from build123d import *

# Parameters (mm, degrees)
BOSS_EXTRUDE1_DEPTH = 40
BOSS_EXTRUDE3_DEPTH = 2.35
BOSS_EXTRUDE4_DEPTH = 2.7
SKETCH7_R           = 5
BOSS_EXTRUDE5_DEPTH = 1
SKETCH8_R           = 2.5
BOSS_EXTRUDE6_DEPTH = 4.6
BOSS_EXTRUDE7_DEPTH = 0.5


with BuildPart() as part:
    # Sketch1 → Boss-Extrude1 (new body)
    with BuildSketch(Plane.XY):
        with BuildLine():
            Line((1.27, 0), (18.68, 0))
            ThreePointArc((18.68, 0), (19.578025612, 0.371974388), (19.95, 1.27))
            Line((19.95, 1.27), (19.95, 36.4))
            Line((19.95, 36.4), (0, 36.4))
            Line((0, 36.4), (0, 1.27))
            ThreePointArc((0, 1.27), (0.371974388, 0.371974388), (1.27, 0))
        make_face()
    extrude(amount=BOSS_EXTRUDE1_DEPTH)

    # Sketch5 → Boss-Extrude3 (add)
    with BuildSketch(Plane(origin=(0, 28, 0), x_dir=(-1, 0, 0), z_dir=(0, -1, 0))):
        with BuildLine():
            Line((0, 0), (0, 7))
            Line((0, 7), (-3.470401751, 7))
            Line((-3.470401751, 7), (-2.98203275, 5.390690104))
            ThreePointArc((-2.98203275, 5.390690104), (-4.95, 2.05), (-6.91796725, 5.390690104))
            Line((-6.91796725, 5.390690104), (-6.429598249, 7))
            Line((-6.429598249, 7), (-13.370401751, 7))
            Line((-13.370401751, 7), (-12.88203275, 5.390690104))
            ThreePointArc((-12.88203275, 5.390690104), (-14.85, 2.05), (-16.81796725, 5.390690104))
            Line((-16.81796725, 5.390690104), (-16.329598249, 7))
            Line((-16.329598249, 7), (-19.8, 7))
            Line((-19.8, 7), (-19.8, 0))
            Line((-19.8, 0), (0, 0))
        make_face()
        with BuildLine():
            Line((-16.329598249, -47), (-16.81796725, -45.390690104))
            ThreePointArc((-16.81796725, -45.390690104), (-14.85, -42.05), (-12.88203275, -45.390690104))
            Line((-12.88203275, -45.390690104), (-13.370401751, -47))
            Line((-13.370401751, -47), (-6.429598249, -47))
            Line((-6.429598249, -47), (-6.91796725, -45.390690104))
            ThreePointArc((-6.91796725, -45.390690104), (-4.95, -42.05), (-2.98203275, -45.390690104))
            Line((-2.98203275, -45.390690104), (-3.470401751, -47))
            Line((-3.470401751, -47), (0, -47))
            Line((0, -47), (0, -40))
            Line((0, -40), (-19.8, -40))
            Line((-19.8, -40), (-19.8, -47))
            Line((-19.8, -47), (-16.329598249, -47))
        make_face()
    extrude(amount=-BOSS_EXTRUDE3_DEPTH)

    # Sketch6 → Boss-Extrude4 (add)
    with BuildSketch(Plane(origin=(0, 36.4, 0), x_dir=(1, 0, 0), z_dir=(0, 1, 0))):
        with BuildLine():
            Line((19.95, -3.7), (19.95, -40))
            Line((19.95, -40), (0, -40))
            Line((0, -40), (0, -3.7))
            Line((0, -3.7), (8.380131585, -3.7))
            ThreePointArc((8.380131585, -3.7), (9.9, -3), (11.419868415, -3.7))
            Line((11.419868415, -3.7), (19.95, -3.7))
        make_face()
    extrude(amount=BOSS_EXTRUDE4_DEPTH)

    # Sketch7 → Boss-Extrude5 (add)
    with BuildSketch(Plane(origin=(0, 39.1, 0), x_dir=(1, 0, 0), z_dir=(0, 1, 0))):
        with Locations((9.95, -30)):
            Circle(SKETCH7_R)
    extrude(amount=BOSS_EXTRUDE5_DEPTH)

    # Sketch8 → Boss-Extrude6 (add)
    with BuildSketch(Plane(origin=(0, 40.1, 0), x_dir=(1, 0, 0), z_dir=(0, 1, 0))):
        with Locations((9.95, -30)):
            Circle(SKETCH8_R)
    extrude(amount=BOSS_EXTRUDE6_DEPTH)

    # Sketch9 → Boss-Extrude7 (add, symmetric)
    with BuildSketch(Plane.ZY.offset(-9.9)):
        Polygon((47, 30.35), (40, 34.1), (40, 30.35), align=None)
    extrude(amount=BOSS_EXTRUDE7_DEPTH, both=True)


solid = part.part
Verification items for the finished model (mm, model axes). A direction names the side the tool comes from. Give positions to 0.01 mm unless a question says otherwise; leave off trailing zeros. Order: outer loops, then holes, each group sorted by start corner. A loop starts at its lowest first (then second) coordinate and runs counter-clockwise, first axis right, second up. Notation, with made-up numbers: M 70.25,36 L 80.25,36 A14 ccw 80.25,63 Z; hole C 44.5,-0.75 d2. An arc over 180 degrees is marked long. Answer as a JSON object with one key per item and string values. Group by question number.
1) Access from +Z, -Z, +X, -X, +Y, -Y to the whole of each face (thin tool, end or side, straight path). Record for faces 1 (the face through (4.8, 30.35, 41.9)), 2 (the face through (16.58, 29.16, -6.18)), 3 (the face through (10.4, 31, 42)).
2) Cross-section at C-C (y = 13.5). Enter the section's corners in (x, z).
3) Cross-section at D-D (z = 44.3). Enter the section's corners in (x, y), then the cut area to 3 significant figures.
4) Cross-section at B-B (z = 30). Enter the section's corners in (x, y).
5) Cross-section at A-A (z = -4.3). Enter the section's corners in (x, y).
6) Scan lines: line 1 along X through (y, z) = (29.5, 44.3); line 2 along Z through (x, y) = (14.85, 28.95); line 3 along Z through (x, y) = (4.5, 36.5). Record each from-to range of solid material in increasing order. Write a range as [from, to].
7) Depth check by flat-ended pin: pin 1 Ø6 at (x, z) = (4.95, -4.3) entering from +Y; pin 2 Ø1.5 at (x, y) = (7, 23) entering from +Z; pin 3 Ø2 at (x, z) = (7, -4.5) entering from -Y. Enter the tip coordinate at first touch or a pass-through.
8) Mould release check, pull along Z, two halves, no side actions. Record for faces 4 (the face through (18, 29, 47)), 5 (the face through (18, 29, -7)), 6 (the face through (4.88, 29.16, -2.05)), 7 (the face through (8.87, 39.59, 34.88)): released by +Z, released by -Z, zero draft, split by the parting line, or undercut.
Result sheet:
{
 "1": {"face 1": "+Z, -X, +Y", "face 2": "+Y, -Y", "face 3": "+Z, +X, +Y"},
 "2": {"outline": "M 0,0 L 19.95,0 L 19.95,40 L 0,40 Z"},
 "3": {"outline": "M 0,28 L 2.7,28 L 2.7,30.35 L 0,30.35 Z; M 7.2,28 L 12.6,28 L 12.6,30.35 L 10.4,30.35 L 10.4,31.8 L 9.4,31.8 L 9.4,30.35 L 7.2,30.35 Z; M 17.1,28 L 19.8,28 L 19.8,30.35 L 17.1,30.35 Z", "area": "26.8 mm2"},
 "4": {"outline": "M 0,1.27 A1.27 ccw 1.27,0 L 18.68,0 A1.27 ccw 19.95,1.27 L 19.95,39.1 L 14.95,39.1 L 14.95,40.1 L 12.45,40.1 L 12.45,44.7 L 7.45,44.7 L 7.45,40.1 L 4.95,40.1 L 4.95,39.1 L 0,39.1 Z"},
 "5": {"outline": "M 0,28 L 2.7,28 L 2.7,30.35 L 0,30.35 Z; M 7.2,28 L 12.6,28 L 12.6,30.35 L 7.2,30.35 Z; M 17.1,28 L 19.8,28 L 19.8,30.35 L 17.1,30.35 Z"},
 "6": {"line 1": "x = [0, 2.7], [7.2, 12.6], [17.1, 19.8]", "line 2": "z = [-2.05, 42.05]", "line 3": "z = [3.7, 40]"},
 "7": {"pin 1": "stops at y = 30.35", "pin 2": "stops at z = 40", "pin 3": "stops at y = 28"},
 "8": {"face 4": "released by +Z", "face 5": "released by -Z", "face 6": "undercut", "face 7": "split by the parting line"}
}
